Part print with two shaded views. Sizes in mm from the minimum x, y, z corner. Coordinates: 2 decimals unless noted, no trailing zeros. Order: outer loops, then holes, each group sorted by start corner. A loop starts at its lowest first (then second) coordinate and runs counter-clockwise, first axis right, second up. Notation, with made-up numbers: M 30,61.5 L 88,61.5 A24 cw 88,80.5 Z; hole C -33.75,-33 d7. An arc over 180 degrees is marked long. Answer in a Markdown table with one row per item. Add a question column.
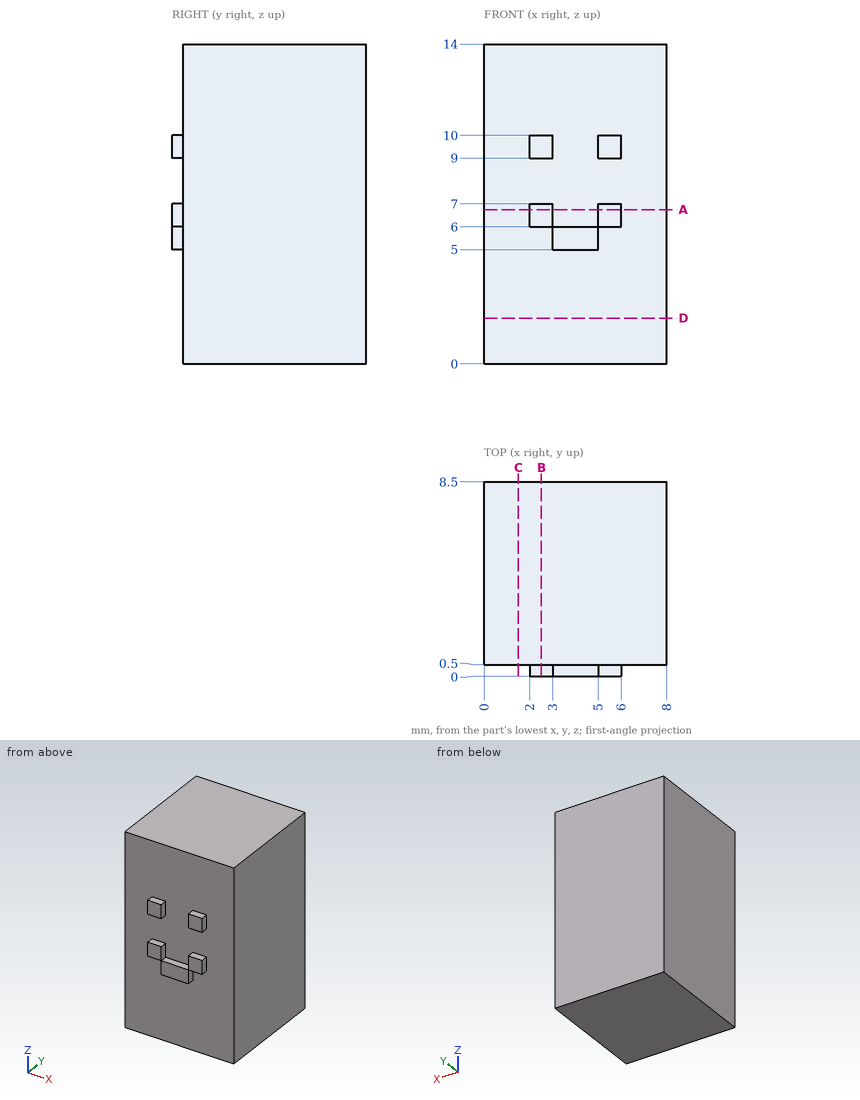
(1) Slice it at A-A (z = 6.75). List the corners of the cut face in (x, y).
(2) Slice it at C-C (x = 1.5). List the corners of the cut face in (y, z).
(3) Drop flat-ended pins along their axis: P1, Ø0.6, axis at y = 0, z = 9.5, coming from the -X side; P2, Ø1.5, axis at x = 4.5, z = 1.5, coming from the -Y side; P3, Ø0.6, axis at x = 2.5, y = 0, coming from the -Z side. Give the stop position or say it passes through.
(4) Slice it at D-D (z = 2). List the corners of the cut face in (x, y), and give its area (3 significant figures).
(5) Slice it at B-B (x = 2.5). List the corners of the cut face in (y, z), and give its area (3 significant figures).
(6) Wall check: line 1 (Y direction, x = 7, z = 12.5). Give the ranges that are in metal, low to high.
Computed:
| question | item | result |
|---|---|---|
| 1 | outline | M 0,0.5 L 2,0.5 L 2,0 L 3,0 L 3,0.5 L 5,0.5 L 5,0 L 6,0 L 6,0.5 L 8,0.5 L 8,8.5 L 0,8.5 Z |
| 2 | outline | M 0.5,0 L 8.5,0 L 8.5,14 L 0.5,14 Z |
| 3 | P1 | stops at x = 2 |
| 3 | P2 | stops at y = 0.5 |
| 3 | P3 | stops at z = 6 |
| 4 | outline | M 0,0.5 L 8,0.5 L 8,8.5 L 0,8.5 Z |
| 4 | area | 64.0 mm^2 |
| 5 | outline | M 0,6 L 0.5,6 L 0.5,0 L 8.5,0 L 8.5,14 L 0.5,14 L 0.5,10 L 0,10 L 0,9 L 0.5,9 L 0.5,7 L 0,7 Z |
| 5 | area | 113 mm^2 |
| 6 | line 1 | y = 0.5 to 8.5 |
